For this review, take the finished solid that the model builds, in its own axes (mm). Coordinates: 2 decimals unless noted, no trailing zeros. Write each loop counter-clockwise with the first axis right and the second up, starting at its lowest first coordinate (ties: lowest second). Pieces come first, ordered by that corner, then holes. Notation, with made-up numbers: M 71,85 L 130,85 A21 ccw 130,122 Z; hole C -25.5,22 d8. An arc over 180 degrees is marked long. One line per question, with ' | ' between items.
from build123d import *

# Parameters (mm, degrees)
SKETCH1_R               = 17
BOSS_EXTRUDE1_DEPTH     = 4.4
CAVITY1_OUTLINE_R       = 3.15
CAVITY1_DEPTH           = 3.283595969
CAVITY1_START           = 1.183595969
CAVITY1_2_OUTLINE_R     = 3.15
CAVITY1_2_OUTLINE_R_2   = 1.575
CAVITY1_2_DEPTH         = 2.1
SKETCH9_R               = 12.8
BOSS_EXTRUDE3_DEPTH     = 5.6
BOSS_EXTRUDE8_DEPTH     = 8
SKETCH2_R               = 0.6
CUT_EXTRUDE1_DEPTH      = 31.033314835
CIRPATTERN1_COUNT       = 6
CUT_EXTRUDE2_START      = -3.283596
SKETCH3_R               = 4.596048158
CUT_EXTRUDE2_DEPTH      = 3.283596
CUT_EXTRUDE3_DEPTH      = 31.033314835
CUT_EXTRUDE3_DEPTH_BACK = 4
SKETCH4_R               = 4
SKETCH6_R               = 1.8
CUT_EXTRUDE4_DEPTH      = 31.033314835
SKETCH12_4_OUTSIDE_W    = 46.268
SKETCH12_4_OUTSIDE_H    = 46.268
CUT_EXTRUDE5_DEPTH      = 27.038433133


# Read off the part's stored shape, not the designer's step: Cavity1
with BuildPart() as part:
    # Sketch1 → Boss-Extrude1 (new body)
    with BuildSketch(Plane.XY):
        Circle(SKETCH1_R)
    extrude(amount=BOSS_EXTRUDE1_DEPTH)

    # Cavity1 outline → Cavity1 (cut)
    with BuildSketch(Plane.XY):
        with BuildLine():
            Line((3.9375, 6.819950055), (2.048148228, 15.163776711))
            ThreePointArc((2.048148228, 15.163776711), (0, 16.8), (-2.048148228, 15.163776711))
            Line((-2.048148228, 15.163776711), (-3.9375, 6.819950055))
            Line((-3.9375, 6.819950055), (-12.108141735, 9.355636751))
            ThreePointArc((-12.108141735, 9.355636751), (-14.549226784, 8.4), (-14.156289963, 5.80813996))
            Line((-14.156289963, 5.80813996), (-7.875, 0))
            Line((-7.875, 0), (-14.156289963, -5.80813996))
            ThreePointArc((-14.156289963, -5.80813996), (-14.549226784, -8.4), (-12.108141735, -9.355636751))
            Line((-12.108141735, -9.355636751), (-3.9375, -6.819950055))
            Line((-3.9375, -6.819950055), (-2.048148228, -15.163776711))
            ThreePointArc((-2.048148228, -15.163776711), (0, -16.8), (2.048148228, -15.163776711))
            Line((2.048148228, -15.163776711), (3.9375, -6.819950055))
            Line((3.9375, -6.819950055), (12.108141735, -9.355636751))
            ThreePointArc((12.108141735, -9.355636751), (14.549226784, -8.4), (14.156289963, -5.80813996))
            Line((14.156289963, -5.80813996), (7.875, 0))
            Line((7.875, 0), (14.156289963, 5.80813996))
            ThreePointArc((14.156289963, 5.80813996), (14.549226784, 8.4), (12.108141735, 9.355636751))
            Line((12.108141735, 9.355636751), (3.9375, 6.819950055))
        make_face()
        Circle(CAVITY1_OUTLINE_R, mode=Mode.SUBTRACT)
    extrude(amount=CAVITY1_DEPTH, mode=Mode.SUBTRACT)

    # Cavity1 2 outline → Cavity1 2 (cut)
    with BuildSketch(Plane.XY.offset(CAVITY1_START)):
        Circle(CAVITY1_2_OUTLINE_R)
        Circle(CAVITY1_2_OUTLINE_R_2, mode=Mode.SUBTRACT)
    extrude(amount=CAVITY1_2_DEPTH, mode=Mode.SUBTRACT)

    # Sketch9 → Boss-Extrude3 (add)
    with BuildSketch(Plane.XY.offset(4.4)):
        Circle(SKETCH9_R)
    extrude(amount=BOSS_EXTRUDE3_DEPTH)

    # Sketch12 → Boss-Extrude8 (add)
    with BuildSketch(Plane.XY.offset(10)):
        Polygon((3.9, -6.75499815), (7.8, 0), (3.9, 6.75499815), (-3.9, 6.75499815), (-7.8, 0), (-3.9, -6.75499815), align=None)
    extrude(amount=BOSS_EXTRUDE8_DEPTH)

    # Sketch2 → Cut-Extrude1 (cut, through all)
    with BuildSketch(Plane(origin=(0, 0, 0), x_dir=(-1, 0, 0), z_dir=(0, 0, -1))):
        with Locations(Location((0, 13.5, 0), (0, 0, 180))):
            Circle(SKETCH2_R)
        with Locations(Location((0, 10.5, 0), (0, 0, 180))):
            Circle(SKETCH2_R)
        with Locations(Location((0, 7.5, 0), (0, 0, 180))):
            Circle(SKETCH2_R)
    cut_extrude1 = extrude(amount=-CUT_EXTRUDE1_DEPTH, mode=Mode.SUBTRACT)

    # CirPattern1: Cut-Extrude1 ×6 about axis
    cirpattern1_axis = Axis((0, 0, 0), (0, 0, 1))
    for i in range(1, CIRPATTERN1_COUNT):
        add(cut_extrude1.rotate(cirpattern1_axis, i * 360 / CIRPATTERN1_COUNT), mode=Mode.SUBTRACT)

    # Sketch3 → Cut-Extrude2 (cut)
    with BuildSketch(Plane(origin=(0, 0, 0), x_dir=(-1, 0, 0), z_dir=(0, 0, -1)).offset(CUT_EXTRUDE2_START)):
        Circle(SKETCH3_R)
    extrude(amount=CUT_EXTRUDE2_DEPTH, mode=Mode.SUBTRACT)

    # Sketch4 → Cut-Extrude3 (cut, two sides: drawn at the far end of the back side and taken through both)
    with BuildSketch(Plane.XY.offset(-CUT_EXTRUDE3_DEPTH_BACK)):
        Circle(SKETCH4_R)
    extrude(amount=CUT_EXTRUDE3_DEPTH + CUT_EXTRUDE3_DEPTH_BACK, mode=Mode.SUBTRACT)

    # Sketch6 → Cut-Extrude4 (cut, through all)
    with BuildSketch(Plane(origin=(0, 0, 0), x_dir=(-1, 0, 0), z_dir=(0, 0, -1))):
        with Locations(Location((-7.875, 0, 0), (0, 0, 302.067932294))):
            Circle(SKETCH6_R)
        with Locations(Location((7.875, 0, 0), (0, 0, 42.758730598))):
            Circle(SKETCH6_R)
    extrude(amount=-CUT_EXTRUDE4_DEPTH, mode=Mode.SUBTRACT)

    # Sketch12<4> outside → Cut-Extrude5 (cut, through all)
    with BuildSketch(Plane.XY.offset(10)):
        Rectangle(SKETCH12_4_OUTSIDE_W, SKETCH12_4_OUTSIDE_H)
        Polygon((3.9, -6.75499815), (7.8, 0), (3.9, 6.75499815), (-3.9, 6.75499815), (-7.8, 0), (-3.9, -6.75499815), align=None, mode=Mode.SUBTRACT)
    extrude(amount=-CUT_EXTRUDE5_DEPTH, mode=Mode.SUBTRACT)


solid = part.part
1. Take a section at D-D on x = -4.75. State the section outline as (y, z) points.
Computed values:
outline: M -5.28,3.28 L 5.28,3.28 L 5.28,18 L -5.28,18 Z
2. Draft analysis for pull direction Y (two halves, no side actions). For faces 1 (the cylindrical face through (-0.867, -3.905, 10.539)), 2 (the flat face through (5.389, -4.177, 10.745)), 3 (the flat face through (3, -3, 18)), state which applies: pulls with the +Y half, pulls with the -Y half, needs draft (parallel to the pull), parting line crosses it, or undercut.
Computed values:
face 1: undercut | face 2: pulls with the -Y half | face 3: needs draft
3. Take a section at B-B on x = 0. State the section outline as (y, z) points (3 decimals).
Computed values:
outline: M -6.755,3.284 L -4,3.284 L -4,18 L -6.755,18 Z; M 4,3.284 L 6.755,3.284 L 6.755,18 L 4,18 Z
4. Clearance check with a flat-ended pin moving along its axis: P1, Ø6, axis at y = 4, z = 14, coming from the -X side. State where the tip first meets the part, or that it passes through.
Computed values:
P1: stops at x = -6.92
5. Take a section at A-A on z = 16.5. State the section outline as (x, y) points (3 decimals).
Computed values:
outline: M -6.919,-1.525 L -3.9,-6.755 L 3.9,-6.755 L 6.919,-1.525 A1.8 cw 6.919,1.525 L 3.9,6.755 L -3.9,6.755 L -6.919,1.525 A1.8 cw Z; hole C 0,0 d8
6. Take a section at C-C on y = -2.25. State the section outline as (x, z) points.
Computed values:
outline: M -6.5,3.28 L -3.31,3.28 L -3.31,18 L -6.5,18 Z; M 3.31,3.28 L 6.5,3.28 L 6.5,18 L 3.31,18 Z
7. For line 1 along Y through (x, z) = (0, 9) (3 decimals); line 2 along X through (y, z) = (-3.5, 4.5); line 3 along X through (y, z) = (-2.75, 7.5), list the stretches that pass through material, from the lowest coordinate up.
Computed values:
line 1: y = -6.755 to -4, 4 to 6.755 | line 2: x = -5.78 to -1.94, 1.94 to 5.78 | line 3: x = -6.21 to -2.9, 2.9 to 6.21
